```python
from build123d import *

# Parameters (mm, degrees)
SKETCH_1_W               = 55
SKETCH_1_H               = 44
EXTRUDE_1_DEPTH          = 18
SKETCH_2_R               = 4
CUT_EXTRUDE_1_DEPTH      = 18
HOLE_WIZARD_6_5_6_5_1_D  = 6.5
SKETCH_5_W               = 25
SKETCH_5_H               = 50
CUT_EXTRUDE_2_DEPTH      = 8
SKETCH_6_W               = 47
SKETCH_6_H               = 44
SKETCH_6_R               = 15
EXTRUDE_2_DEPTH          = 5
HOLE_WIZARD_3_2_3_2_1_D  = 3.2
PATTERN_CIRCULAR_1_COUNT = 4
SKETCH_9_W               = 200
SKETCH_9_H               = 100
CUT_EXTRUDE_3_DEPTH      = 1


with BuildPart() as part:
    # Эскиз1 → Бобышка-Вытянуть1 (new body)
    with BuildSketch(Plane.XY):
        Rectangle(SKETCH_1_W, SKETCH_1_H)
    extrude(amount=EXTRUDE_1_DEPTH)

    # Эскиз2 → Вырез-Вытянуть1 (cut)
    with BuildSketch(Plane.XY.offset(18)):
        with Locations((-6, 0)):
            Circle(SKETCH_2_R)
    extrude(amount=-CUT_EXTRUDE_1_DEPTH, mode=Mode.SUBTRACT)

    # Диаметр отверстия Ø6.5 (6.5)1 (through all)
    with Locations(Plane(origin=(0, 22, 0), x_dir=(1, 0, 0), z_dir=(0, 1, 0))):
        with Locations((19.8, -9), (-19.8, -9)):
            Hole(HOLE_WIZARD_6_5_6_5_1_D / 2)

    # Эскиз5 → Вырез-Вытянуть2 (cut)
    with BuildSketch(Plane(origin=(0, 0, 0), x_dir=(-1, 0, 0), z_dir=(0, 0, -1))):
        Rectangle(SKETCH_5_W, SKETCH_5_H)
    extrude(amount=-CUT_EXTRUDE_2_DEPTH, mode=Mode.SUBTRACT)

    # Эскиз6 → Бобышка-Вытянуть2 (add)
    with BuildSketch(Plane.XY.offset(18)):
        with Locations((-51, 0)):
            Rectangle(SKETCH_6_W, SKETCH_6_H)
        with Locations((-51, 0)):
            Circle(SKETCH_6_R, mode=Mode.SUBTRACT)
    extrude(amount=-EXTRUDE_2_DEPTH)

    # Диаметр отверстия Ø3.2 (3.2)1 (through all)
    with Locations(Plane(origin=(0, 0, 13), x_dir=(-1, 0, 0), z_dir=(0, 0, -1))):
        with Locations((35.5, -15.5)):
            hole_wizard_3_2_3_2_1 = Hole(HOLE_WIZARD_3_2_3_2_1_D / 2)

    # Круговой массив1: Диаметр отверстия Ø3.2 (3.2)1 ×4 about axis
    pattern_circular_1_axis = Axis((-51, 0, 0), (0, 0, 1))
    for i in range(1, PATTERN_CIRCULAR_1_COUNT):
        add(hole_wizard_3_2_3_2_1.rotate(pattern_circular_1_axis, i * 360 / PATTERN_CIRCULAR_1_COUNT), mode=Mode.SUBTRACT)

    # Эскиз9 → Вырез-Вытянуть3 (cut)
    with BuildSketch(Plane.XY.offset(18)):
        Rectangle(SKETCH_9_W, SKETCH_9_H)
    extrude(amount=-CUT_EXTRUDE_3_DEPTH, mode=Mode.SUBTRACT)


solid = part.part
```
Could you check a few things on this model? Use its own coordinates, in mm. A direction names the side the tool comes from. Coordinates: 2 decimals unless noted, no trailing zeros. Order: outer loops, then holes, each group sorted by start corner. A loop starts at its lowest first (then second) coordinate and runs counter-clockwise, first axis right, second up. Notation, with made-up numbers: M 68,20.5 L 73,20.5 A15 cw 73,42.5 Z; hole C -21,4.25 d5. An arc over 180 degrees is marked long. Use one line per item in the form item = value. Start each with the question number.
1. Please list where these lines run through material, in increasing order: line 1 (X direction, y = 20.5, z = 9); line 2 (Y direction, x = -66.5, z = 14.85); line 3 (X direction, y = 13, z = 6.25).
2. For pin 1 (3.5 mm diameter, centred on x = -35.5, y = -15.5, fed in from -Z); pin 2 (6.5 mm diameter, centred on y = 5.5, z = 2.5, fed in from -X); pin 3 (4 mm diameter, centred on x = -7, y = 15, fed in from -Z), each with a flat end and sliding along its axis, tell me the tip position at first contact or that it passes through.
3. Suppose I cut it at B-B on y = 0. Write out the boundary of the cut face in (x, z), then the cut area to 3 significant figures.
4. On a 3-axis mill with a long thin cutter (end or side, diameter ignored), from which of +Z, -Z, +X, -X, +Y, -Y can I reach the whole of each face in a straight line? I mean faces 1 (the flat face through (-20, 0, 0)), 2 (the flat face through (12.5, 0, 4)), 3 (the flat face through (-46, 15, 13)). Say none if no direction works.
5. Suppose I cut it at D-D on y = 10. Write out the boundary of the cut face in (x, z).
6. Suppose I cut it at A-A on z = 9. Write out the boundary of the cut face in (x, y).
7. We'd pull the mould along Y, two halves only. Please class faces 4 (the flat face through (-13, -22, 11)), 5 (the flat face through (-24, 0, 17)), 6 (the cylindrical face through (-6.867, -3.905, 12.563)): +Y half, -Y half, draft (parallel to the pull), parting line (faces both ways), or undercut.
8. Suppose I cut it at C-C on x = -51. Write out the boundary of the cut face in (y, z), then the cut area to 3 significant figures.
Geometry says:
q1.line_1 = -27.5 to -23.05, -16.55 to 16.55, 23.05 to 27.5
q1.line_2 = -22 to -17.1, -13.9 to 13.9, 17.1 to 22
q1.line_3 = -27.5 to -21.53, -18.07 to -12.5, 12.5 to 18.07, 21.53 to 27.5
q2.pin_1 = 13
q2.pin_2 = -27.5
q2.pin_3 = 8
q3.outline = M -74.5,13 L -66,13 L -66,17 L -74.5,17 Z; M -36,13 L -27.5,13 L -27.5,0 L -12.5,0 L -12.5,8 L -10,8 L -10,17 L -36,17 Z; M -2,8 L 12.5,8 L 12.5,0 L 27.5,0 L 27.5,17 L -2,17 Z; hole C -19.8,9 d6.5; hole C 19.8,9 d6.5
q3.area = 665 mm^2
q4.face_1 = -Z, +X, -X, +Y, -Y
q4.face_2 = -Z, +Y, -Y
q4.face_3 = -Z, -X, +Y, -Y
q5.outline = M -74.5,13 L -62.18,13 L -62.18,17 L -74.5,17 Z; M -39.82,13 L -27.5,13 L -27.5,0 L -12.5,0 L -12.5,8 L 12.5,8 L 12.5,0 L 27.5,0 L 27.5,17 L -39.82,17 Z; hole C -19.8,9 d6.5; hole C 19.8,9 d6.5
q6.outline = M -27.5,-22 L -23.05,-22 L -23.05,22 L -27.5,22 Z; M -16.55,-22 L 16.55,-22 L 16.55,22 L -16.55,22 Z; M 23.05,-22 L 27.5,-22 L 27.5,22 L 23.05,22 Z; hole C -6,0 d8
q7.face_4 = -Y half
q7.face_5 = draft
q7.face_6 = undercut
q8.outline = M -22,13 L -15,13 L -15,17 L -22,17 Z; M 15,13 L 22,13 L 22,17 L 15,17 Z
q8.area = 56.0 mm^2
